```python
from build123d import *

# Parameters (mm, degrees)
F1_DEPTH = 200
F2_SIZE  = 1
F3_SIZE  = 3


with BuildPart() as f1:
    # F0 (on Front) → F1 (new body)
    with BuildSketch(Plane.XZ):
        Polygon((0, 20), (0, 0), (20, 0), (20, 3), (10, 3), (10, 10), (3, 10), (3, 20), align=None)
    extrude(amount=F1_DEPTH)

    # F2
    f2_edges = [f1.edges().sort_by_distance(p)[0] for p in [
        (0, -100, 20),
        (3, -100, 20),
        (20, -100, 3),
        (20, -100, 0),
        (0, -100, 0),
    ]]
    chamfer(f2_edges, length=F2_SIZE)

    # F3
    f3_edges = [f1.edges().sort_by_distance(p)[0] for p in [
        (10, -100, 10),
    ]]
    chamfer(f3_edges, length=F3_SIZE)


solid = f1.part
```
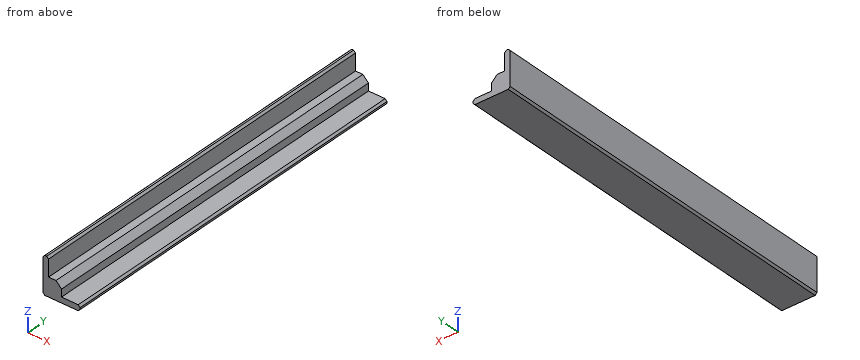
Geometry check sheet. Reference: the model listing, model coordinates, mm. Coordinates: 2 decimals unless noted, no trailing zeros. Order: outer loops, then holes, each group sorted by start corner. A loop starts at its lowest first (then second) coordinate and runs counter-clockwise, first axis right, second up.
Q1. Sectioned sample at C-C on z = 5.25. Record the cut outline in (x, y), and give its area (3 significant figures).
Reply:
outline: (0, -200) - (10, -200) - (10, 0) - (0, 0) - close
area: 2,000 mm2
Q2. Sectioned sample at A-A on y = -177.5. Record the cut outline in (x, z), and give its area (3 significant figures).
Reply:
outline: (0, 1) - (1, 0) - (19, 0) - (20, 1) - (20, 2) - (19, 3) - (10, 3) - (10, 7) - (7, 10) - (3, 10) - (3, 19) - (2, 20) - (1, 20) - (0, 19) - close
area: 153 mm2
Q3. Depth check by flat-ended pin: pin 1 Ø12 at (y, z) = (-170.5, 9.5) entering from +X; pin 2 Ø7 at (x, y) = (12.5, -112.5) entering from +Z; pin 3 Ø6 at (y, z) = (-23, 17.5) entering from +X. Enter the tip coordinate at first touch or a pass-through.
Reply:
pin 1: stops at x = 10
pin 2: stops at z = 8
pin 3: stops at x = 3
Q4. Sectioned sample at B-B on x = 13.5. Record the cut outline in (y, z).
Reply:
outline: (-200, 0) - (0, 0) - (0, 3) - (-200, 3) - close
Q5. Thickness scan on probe 1 along Z at (x, y) = (17.25, -134); probe 2 along Z at (x, y) = (5.25, -165.5). Record the ranges inside material, lowest first.
Reply:
probe 1: z = 0 to 3
probe 2: z = 0 to 10
